Autodesk Inventor part; units mm, degrees
ref_plane "YZ Plane" through (0, 0, 0) normal (1, 0, 0) x (0, 1, 0)
ref_plane "XZ Plane" through (0, 0, 0) normal (0, 1, 0) x (-1, 0, 0)
ref_plane "XY Plane" through (0, 0, 0) normal (0, 0, 1) x (1, 0, 0)
sketch "Sketch1" plane through (0, 0, 0) normal (1, 0, 0) x (0, 1, 0)
  circle A0 centre (0, 0) radius 3
  line L0 (6.4648, 15) -> (-155, 15)
  line L1 (-155, 15) -> (-155, -15)
  line L2 (-155, -15) -> (-15.0845, -15)
  line L3 (15, -15) -> (15, 15)
  line L4 (-9.3985, -19.0843) -> (16.2364, -95.1689)
  line L5 (16.2364, -95.1689) -> (44.6661, -85.5902)
  line L6 (44.6661, -85.5902) -> (12.1507, 10.9157)
  line L7 (9.5442, 18.6521) -> (-18.8856, 9.0734)
  arc A1 (-9.3985, -19.0843) -> (-15.0845, -15) centre (-15.0845, -21) ccw
  arc A2 (12.1507, 10.9157) -> (6.4648, 15) centre (6.4648, 9) ccw
  circle A3 centre (-140, 0) radius 10
  circle A4 centre (-140, 0) radius 3
  circle A5 centre (25.6619, -76.1647) radius 10
  dimension "d0" = 6
  dimension "d1" = 170
  dimension "d2" = 30
  dimension "d3" = 110
  dimension "d6" = 108.62
  dimension "d7" = 15
  dimension "d8" = 15
  dimension "d9" = 6
  dimension "d10" = 20
  dimension "d11" = 6
  dimension "d12" = 15
  dimension "d13" = 20
extrude "Extrusion1" add sketch "Sketch1" along normal blind 10 contours A2 L6 L5 L4 A1 L2 L1 L0
properties part number "bogie1"
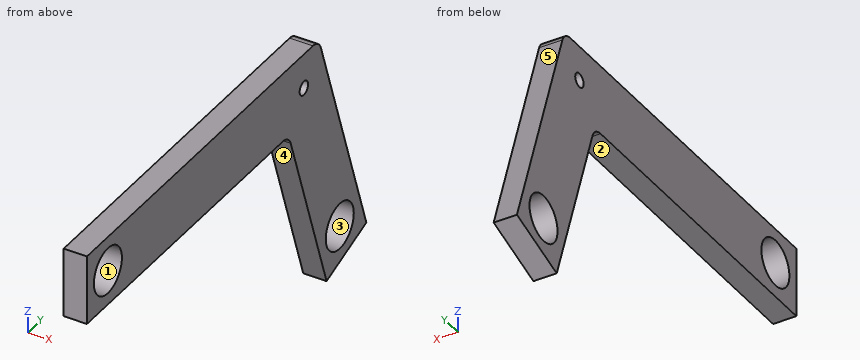
Work out the finished part from the listing and answer in its coordinate system (mm). Face numbers are marked on the shaded views. A direction names the side the tool comes from. Coordinates: 2 decimals unless noted, no trailing zeros. Write each loop counter-clockwise with the first axis right and the second up, starting at its lowest first coordinate (ties: lowest second). Pieces come first, ordered by that corner, then holes.
1. For the marked faces 1 and 2, determine the directions among +Z, -Z, +X, -X, +Y, -Y from which every point of the face is accessible in a straight line to the end or side of a thin tool.
Results list:
face 1: +X, -X
face 2: -Z, +X, -X, -Y
2. Flat-ended cylindrical pins translate along their axes: pin 1 (6 mm diameter, centred on x = 6, z = -74.5, fed in from +Y); pin 2 (4 mm diameter, centred on x = 6.5, z = 0, fed in from +Y); pin 3 (6 mm diameter, centred on x = 2, y = -36.5, fed in from -Z). Find the tip coordinate at first contact, or state that the pin passes through.
Results list:
pin 1: stops at y = 41.94
pin 2: stops at y = 16.5
pin 3: stops at z = -15
3. The part is cut by section B-B, the plane z = 0. Write down the section's boundary in (x, y).
Results list:
outline: (0, -155) - (10, -155) - (10, -150) - (0, -150) - close; (0, -130) - (10, -130) - (10, -3) - (0, -3) - close; (0, 3) - (10, 3) - (10, 15.83) - (0, 15.83) - close
4. The part is cut by section A-A, the plane y = -140. Write down the section's boundary in (x, z), and give its area (3 significant figures).
Results list:
outline: (0, -15) - (10, -15) - (10, -10) - (0, -10) - close; (0, 10) - (10, 10) - (10, 15) - (0, 15) - close
area: 100 mm2
5. For a pull along Y with two mould halves and no side action, classify the marked faces 3, 4 and 5 as +Y half, -Y half, draft (parallel to the pull), parting line (faces both ways), or undercut.
Results list:
face 3: undercut
face 4: -Y half
face 5: +Y half
6. The part is cut by section C-C, the plane x = 8.25. Write down the section's boundary in (y, z), and give its area (3 significant figures).
Results list:
outline: (-155, -15) - (-15.08, -15) arc R6 cw to (-9.4, -19.08) - (16.24, -95.17) - (44.67, -85.59) - (12.15, 10.92) arc R6 ccw to (6.46, 15) - (-155, 15) - close; hole circle Ø20 at (-140, 0); hole circle Ø6 at (0, 0); hole circle Ø20 at (25.66, -76.16)
area: 6,850 mm2
7. The part is cut by section D-D, the plane y = 0. Write down the section's boundary in (x, z), and give its area (3 significant figures).
Results list:
outline: (0, -46.98) - (10, -46.98) - (10, -3) - (0, -3) - close; (0, 3) - (10, 3) - (10, 15) - (0, 15) - close
area: 560 mm2
8. Consider line 1 along Z through (x, y) = (5.25, -140); line 2 along Z through (x, y) = (4, -142); line 3 along Z through (x, y) = (7.25, -97). Determine where each line is inside the solid, lowest interval first.
Results list:
line 1: z = -15 to -10, 10 to 15
line 2: z = -15 to -9.8, 9.8 to 15
line 3: z = -15 to 15
